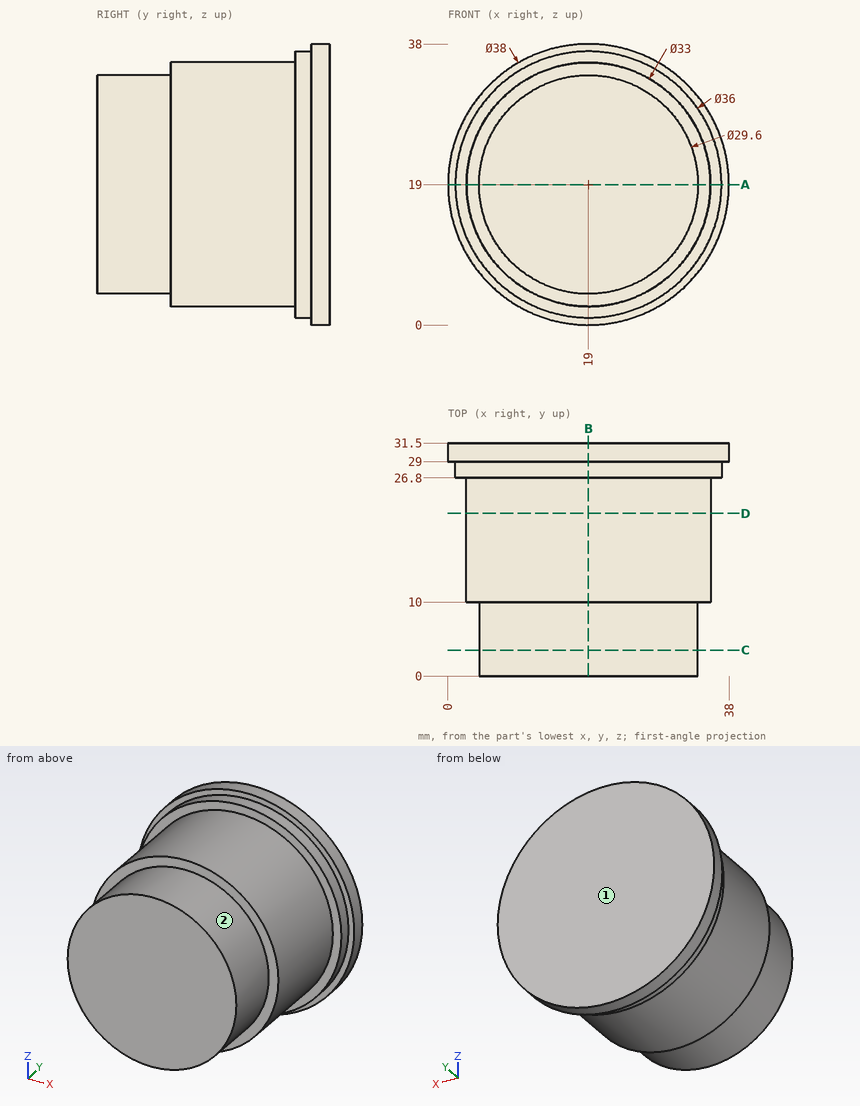
The figure shows three views and two pictorial views of one solid part (mm, origin at its lowest corner). Answer the questions. A direction names the side the tool comes from. Coordinates: 2 decimals unless noted, no trailing zeros. Write each loop counter-clockwise with the first axis right and the second up, starting at its lowest first coordinate (ties: lowest second). Pieces come first, ordered by that corner, then holes.
1. The part is cut by section D-D, the plane y = 22. Write down the section's boundary in (x, z).
Results list:
outline: circle Ø33 at (19, 19)
2. Flat-ended cylindrical pins translate along their axes: pin 1 (1.5 mm diameter, centred on x = 27.5, y = 26, fed in from -Z); pin 2 (2 mm diameter, centred on x = 19, y = 5, fed in from +Z); pin 3 (3 mm diameter, centred on x = 30.5, z = 6, fed in from -Y). Find the tip coordinate at first contact, or state that the pin passes through.
Results list:
pin 1: stops at z = 4.43
pin 2: stops at z = 33.8
pin 3: stops at y = 10
3. Consider line 1 along Z through (x, y) = (19, 17); line 2 along Y through (x, z) = (30, 32.5); line 3 along Y through (x, z) = (27, 5.5). Determine where each line is inside the solid, lowest interval first.
Results list:
line 1: z = 2.5 to 35.5
line 2: y = 26.8 to 31.5
line 3: y = 10 to 31.5
4. The part is cut by section C-C, the plane y = 3.5. Write down the section's boundary in (x, z), and give its area (3 significant figures).
Results list:
outline: circle Ø29.6 at (19, 19)
area: 688 mm2
5. For the marked faces 1 and 2, determine the directions among +Z, -Z, +X, -X, +Y, -Y from which every point of the face is accessible in a straight line to the end or side of a thin tool.
Results list:
face 1: +Z, -Z, +X, -X, +Y
face 2: -Y
6. The part is cut by section A-A, the plane z = 19. Write down the section's boundary in (x, y).
Results list:
outline: (0, 29) - (1, 29) - (1, 26.8) - (2.5, 26.8) - (2.5, 10) - (4.2, 10) - (4.2, 0) - (33.8, 0) - (33.8, 10) - (35.5, 10) - (35.5, 26.8) - (37, 26.8) - (37, 29) - (38, 29) - (38, 31.5) - (0, 31.5) - close
7. The part is cut by section B-B, the plane x = 19. Write down the section's boundary in (y, z).
Results list:
outline: (0, 4.2) - (10, 4.2) - (10, 2.5) - (26.8, 2.5) - (26.8, 1) - (29, 1) - (29, 0) - (31.5, 0) - (31.5, 38) - (29, 38) - (29, 37) - (26.8, 37) - (26.8, 35.5) - (10, 35.5) - (10, 33.8) - (0, 33.8) - close
